```python
from build123d import *

# Parameters (mm, degrees)
SKETCH1_R           = 20
SKETCH1_R_2         = 18
BOSS_EXTRUDE1_DEPTH = 7.75
BOSS_EXTRUDE2_START = -4
SKETCH2_R           = 18
BOSS_EXTRUDE2_DEPTH = 4
CUT_EXTRUDE1_DEPTH  = 1.5
SKETCH4_R           = 1
CUT_EXTRUDE2_DEPTH  = 1.5
SKETCH5_W           = 18
SKETCH5_H           = 38
SKETCH5_W_2         = 13.7
SKETCH5_H_2         = 23.25
BOSS_EXTRUDE3_DEPTH = 4
SKETCH6_R           = 18
BOSS_EXTRUDE4_DEPTH = 2
SKETCH7_R           = 0.5
CUT_EXTRUDE3_DEPTH  = 3
FILLET1_R           = 5


with BuildPart() as part:
    # Sketch1 → Boss-Extrude1 (new body)
    with BuildSketch(Plane(origin=(0, 0, 0), x_dir=(1, 0, 0), z_dir=(0, 1, 0))):
        with Locations(Location((0, 0, 0), (0, 0, 270))):
            Circle(SKETCH1_R)
        with Locations(Location((0, 0, 0), (0, 0, 270))):
            Circle(SKETCH1_R_2, mode=Mode.SUBTRACT)
    extrude(amount=BOSS_EXTRUDE1_DEPTH)

    # Sketch2 → Boss-Extrude2 (add)
    with BuildSketch(Plane(origin=(0, 7.75, 0), x_dir=(1, 0, 0), z_dir=(0, 1, 0)).offset(BOSS_EXTRUDE2_START)):
        with Locations(Location((0, 0, 0), (0, 0, 270))):
            Circle(SKETCH2_R)
    extrude(amount=BOSS_EXTRUDE2_DEPTH)

    # Sketch3 → Cut-Extrude1 (cut)
    with BuildSketch(Plane(origin=(0, 7.75, 0), x_dir=(1, 0, 0), z_dir=(0, 1, 0))):
        with BuildLine():
            Line((-2.4, 2.881405907), (-2, 14.064254381))
            ThreePointArc((-2, 14.064254381), (0, 16.064254381), (2, 14.064254381))
            Line((2, 14.064254381), (2.4, 2.881405907))
            ThreePointArc((2.4, 2.881405907), (0, -3.75), (-2.4, 2.881405907))
        make_face()
    extrude(amount=-CUT_EXTRUDE1_DEPTH, mode=Mode.SUBTRACT)

    # Sketch4 → Cut-Extrude2 (cut)
    with BuildSketch(Plane(origin=(0, 6.25, 0), x_dir=(1, 0, 0), z_dir=(0, 1, 0))):
        with Locations(Location((0, 0, 0), (0, 0, 270))):
            Circle(SKETCH4_R)
    extrude(amount=-CUT_EXTRUDE2_DEPTH, mode=Mode.SUBTRACT)



with BuildPart() as body_2:
    # Sketch5 → Boss-Extrude3 (new body)
    with BuildSketch(Plane(origin=(11.45, 0, 0), x_dir=(0, 0, -1), z_dir=(1, 0, 0))):
        with Locations((0, -19)):
            Rectangle(SKETCH5_W, SKETCH5_H)
        with Locations((0, -17.375)):
            Rectangle(SKETCH5_W_2, SKETCH5_H_2, mode=Mode.SUBTRACT)
    extrude(amount=BOSS_EXTRUDE3_DEPTH)


with BuildPart() as part_1:
    add(part.part)

    add(body_2.part)  # Boss-Extrude4 merges body 2
    # Sketch6 → Boss-Extrude4 (add)
    with BuildSketch(Plane.XZ):
        with Locations(Location((0, 0, 0), (0, 0, 270))):
            Circle(SKETCH6_R)
    extrude(amount=-BOSS_EXTRUDE4_DEPTH)

    # Sketch7 → Cut-Extrude3 (cut)
    with BuildSketch(Plane.ZY.offset(-11.45)):
        with Locations((0, -30.85)):
            Circle(SKETCH7_R)
        with Locations((0, -3.25)):
            Circle(SKETCH7_R)
    extrude(amount=-CUT_EXTRUDE3_DEPTH, mode=Mode.SUBTRACT)

    # Fillet1
    fillet1_edges = [part_1.edges().sort_by_distance(p)[0] for p in [
        (13.45, -38, 9),
        (13.45, -38, -9),
    ]]
    fillet(fillet1_edges, radius=FILLET1_R)


solid = part_1.part
```
Check sheet for the modelled part. Datum: model origin and axes. Units: mm. A direction names the side the tool comes from. Coordinates: 2 decimals unless noted, no trailing zeros. Write each loop counter-clockwise with the first axis right and the second up, starting at its lowest first coordinate (ties: lowest second). Pieces come first, ordered by that corner, then holes. Notation, with made-up numbers: (-16, 36) -> (16, 36) arc R24 ccw to (16, 46) -> close; hole circle Ø10 at (-17.5, 15). An arc over 180 degrees is marked (long way). Use a Markdown table: item, result.
1. Release check for a two-part mould opening along Z. For faces 1 (the flat face through (0, 6.25, -6)), 2 (the flat face through (0, 7.75, 4)), 3 (the cylindrical face through (-19.524, 3.821, -4.336)) record: pulls with the +Z half, pulls with the -Z half, needs draft (parallel to the pull), parting line crosses it, or undercut.
Reported:
| item | result |
|---|---|
| face 1 | undercut |
| face 2 | needs draft |
| face 3 | parting line crosses it |
2. Sectioned sample at C-C (z = 16). Enter the section's corners in (x, y), plus the area to 3 significant figures.
Reported:
| item | result |
|---|---|
| outline | (-12, 0) -> (12, 0) -> (12, 7.75) -> (-12, 7.75) -> close; hole (-8.25, 2) -> (8.25, 2) -> (8.25, 3.75) -> (-8.25, 3.75) -> close |
| area | 157 mm2 |
3. Scan lines: line 1 along Y through (x, z) = (13.15, 0); line 2 along Y through (x, z) = (5, -13); line 3 along X through (y, z) = (5.9, 0). Record each from-to range of solid material in increasing order.
Reported:
| item | result |
|---|---|
| line 1 | y = -38 to -31.35, -30.35 to -29, -5.75 to -3.75, -2.75 to 2, 3.75 to 7.75 |
| line 2 | y = 0 to 2, 3.75 to 7.75 |
| line 3 | x = -20 to -1, 1 to 20 |
4. Sectioned sample at A-A (y = -15). Enter the section's corners in (x, z), plus the area to 3 significant figures.
Reported:
| item | result |
|---|---|
| outline | (11.45, -9) -> (15.45, -9) -> (15.45, -6.85) -> (11.45, -6.85) -> close; (11.45, 6.85) -> (15.45, 6.85) -> (15.45, 9) -> (11.45, 9) -> close |
| area | 17.2 mm2 |
5. Sectioned sample at D-D (y = -32). Enter the section's corners in (x, z).
Reported:
| item | result |
|---|---|
| outline | (11.45, -9) -> (15.45, -9) -> (15.45, 9) -> (11.45, 9) -> close |
6. Sectioned sample at B-B (x = -13). Enter the section's corners in (y, z), plus the area to 3 significant figures.
Reported:
| item | result |
|---|---|
| outline | (0, -15.2) -> (7.75, -15.2) -> (7.75, 15.2) -> (0, 15.2) -> close; hole (2, -12.45) -> (3.75, -12.45) -> (3.75, 12.45) -> (2, 12.45) -> close |
| area | 192 mm2 |
7. Go/stop test with flat-tipped pins: pin 1 Ø6 at (y, z) = (-7, -9.5) entering from -X; pin 2 Ø2 at (x, y) = (13.5, -18) entering from +Z; pin 3 Ø4 at (y, z) = (-20.5, -4) entering from -X; pin 4 Ø20 at (y, z) = (-23.5, 4) entering from +X. Record where each tip stops, or that it passes through.
Reported:
| item | result |
|---|---|
| pin 1 | stops at x = 11.45 |
| pin 2 | stops at z = 9 |
| pin 3 | passes through |
| pin 4 | stops at x = 15.45 |
8. Tool access check on faces 4 (the flat face through (0, 2, 0)), 5 (the flat face through (13, -17, 9)), 6 (the flat face through (0, 4.75, 0)). Record the directions out of +Z, -Z, +X, -X, +Y, -Y that give a thin tool (end or side, any length) a straight path to the whole face; none if there is none.
Reported:
| item | result |
|---|---|
| face 4 | none |
| face 5 | +Z, +X, -X, -Y |
| face 6 | +Y |
